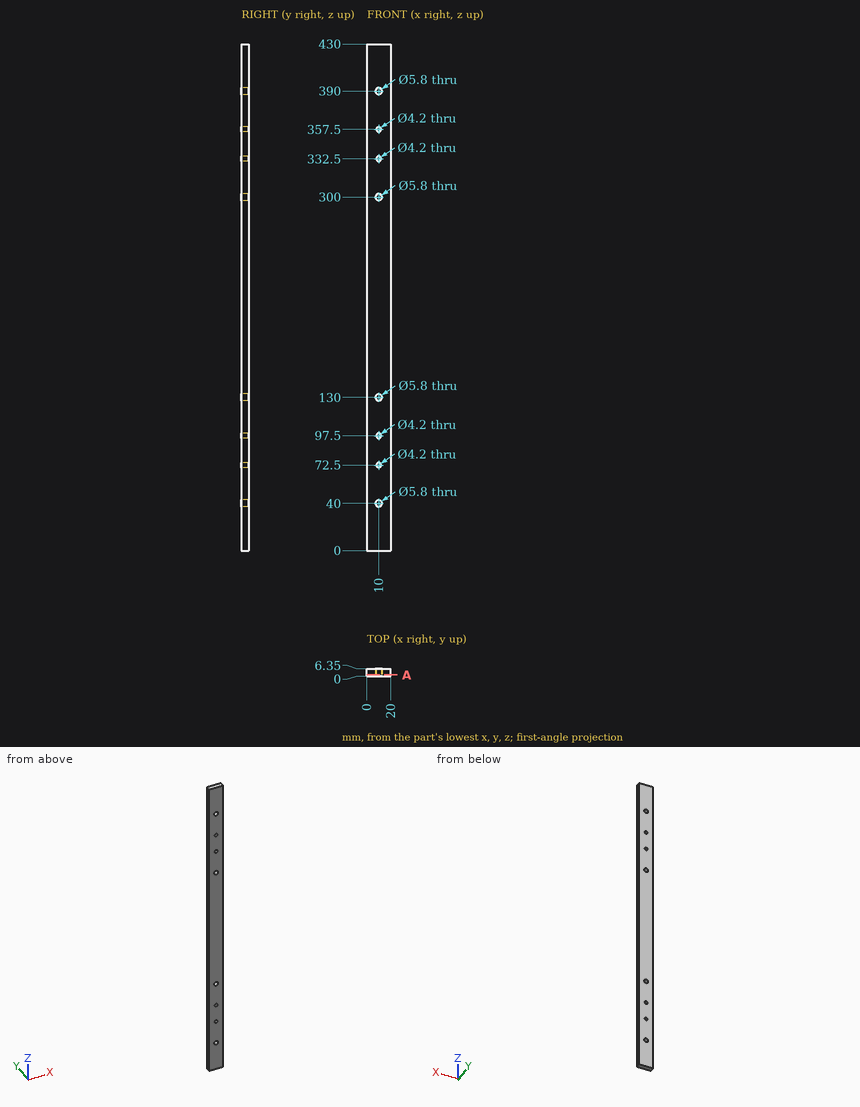
Design review of the part shown in the three views and the two pictorial views. Dimensions are in mm from the part's minimum x, y and z. Round coordinates to 2 decimals unless told otherwise and drop trailing zeros. Use one line per item in the form item = value. Start each with the question number.
Q1. For pin 1 Ø2.5 at (x, z) = (10, 332.5) entering from +Y (3 decimals), flat-tipped, find the tip position at first contact; note if it passes through.
Q2. Wall thickness on line 1 along X through (y, z) = (4.5, 390); line 2 along X through (y, z) = (1.75, 332.5): over which ranges is each line inside the solid? List them lowest first. Write a range as [from, to].
Q3. We need section A-A on y = 1. State how many separate pieces and enclosed holes the cut face has, then the cut area to 3 significant figures.
Calculated:
q1.pin_1 = through
q2.line_1 = [0, 7.1], [12.9, 20]
q2.line_2 = [0, 7.9], [12.1, 20]
q3.separate_pieces = 1
q3.enclosed_holes = 8
q3.area = 8,440 mm²
